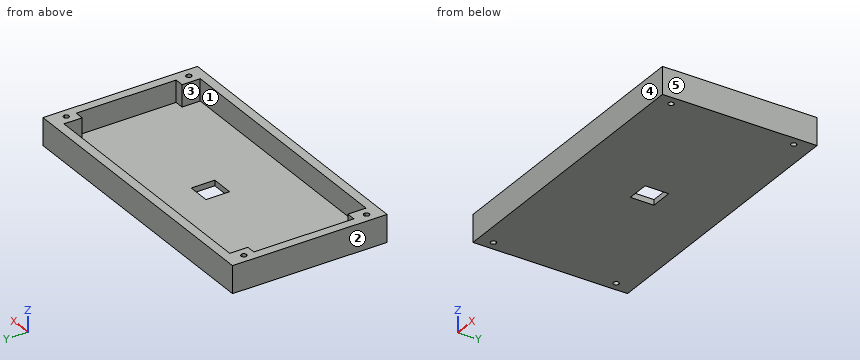
```python
from build123d import *

# Parameters (mm, degrees)
F0_W     = 160
F0_H     = 85
F0_W_2   = 12.5
F0_H_2   = 13
F1_DEPTH = 3
F2_W     = 160
F2_H     = 85
F2_W_2   = 150
F2_H_2   = 75
F3_DEPTH = 12
F5_DEPTH = 12
F6_DEPTH = 15


with BuildPart() as f1:
    # F0 (on Top) → F1 (new body)
    with BuildSketch(Plane.XY):
        with Locations((0, -2.5)):
            Rectangle(F0_W, F0_H)
        Rectangle(F0_W_2, F0_H_2, mode=Mode.SUBTRACT)
    extrude(amount=F1_DEPTH)

    # F2 (on face) → F3 (join)
    with BuildSketch(Plane.XY.offset(3)):
        with Locations((0, -2.5)):
            Rectangle(F2_W, F2_H)
        with Locations((0, -2.5)):
            Rectangle(F2_W_2, F2_H_2, mode=Mode.SUBTRACT)
    extrude(amount=F3_DEPTH)

    # F4 (on face) → F5 (join, through all)
    with BuildSketch(Plane.XY.offset(15)):
        with BuildLine():
            ThreePointArc((75, 29), (73.5, 30.5), (75, 32))
            Line((75, 32), (75, 35))
            Line((75, 35), (70, 35))
            Line((70, 35), (70, 25))
            Line((70, 25), (75, 25))
            Line((75, 25), (75, 29))
        make_face()
        with BuildLine():
            ThreePointArc((-75, 32), (-73.93934, 31.56066), (-73.5, 30.5))
            ThreePointArc((-73.5, 30.5), (-73.93934, 29.43934), (-75, 29))
            Line((-75, 29), (-75, 25))
            Line((-75, 25), (-70, 25))
            Line((-70, 25), (-70, 35))
            Line((-70, 35), (-75, 35))
            Line((-75, 35), (-75, 32))
        make_face()
        with BuildLine():
            ThreePointArc((-75, -35.5), (-73.93934, -35.93934), (-73.5, -37))
            ThreePointArc((-73.5, -37), (-73.93934, -38.06066), (-75, -38.5))
            Line((-75, -38.5), (-75, -40))
            Line((-75, -40), (-70, -40))
            Line((-70, -40), (-70, -30))
            Line((-70, -30), (-75, -30))
            Line((-75, -30), (-75, -35.5))
        make_face()
        with BuildLine():
            ThreePointArc((75, -38.5), (73.5, -37), (75, -35.5))
            Line((75, -35.5), (75, -30))
            Line((75, -30), (70, -30))
            Line((70, -30), (70, -40))
            Line((70, -40), (75, -40))
            Line((75, -40), (75, -38.5))
        make_face()
    extrude(amount=-F5_DEPTH)

    # F4 (on face) → F6 (cut, through all)
    with BuildSketch(Plane.XY.offset(15)):
        with BuildLine():
            ThreePointArc((-75, -38.5), (-73.93934, -38.06066), (-73.5, -37))
            ThreePointArc((-73.5, -37), (-73.93934, -35.93934), (-75, -35.5))
            Line((-75, -35.5), (-75, -38.5))
        make_face()
        with BuildLine():
            Line((-75, -38.5), (-75, -35.5))
            ThreePointArc((-75, -35.5), (-76.5, -37), (-75, -38.5))
        make_face()
        with BuildLine():
            ThreePointArc((75, -38.5), (76.06066, -38.06066), (76.5, -37))
            ThreePointArc((76.5, -37), (76.06066, -35.93934), (75, -35.5))
            Line((75, -35.5), (75, -38.5))
        make_face()
        with BuildLine():
            Line((75, -38.5), (75, -35.5))
            ThreePointArc((75, -35.5), (73.5, -37), (75, -38.5))
        make_face()
        with BuildLine():
            Line((75, 29), (75, 32))
            ThreePointArc((75, 32), (73.5, 30.5), (75, 29))
        make_face()
        with BuildLine():
            ThreePointArc((75, 29), (76.06066, 29.43934), (76.5, 30.5))
            ThreePointArc((76.5, 30.5), (76.06066, 31.56066), (75, 32))
            Line((75, 32), (75, 29))
        make_face()
        with BuildLine():
            ThreePointArc((-75, 29), (-73.93934, 29.43934), (-73.5, 30.5))
            ThreePointArc((-73.5, 30.5), (-73.93934, 31.56066), (-75, 32))
            Line((-75, 32), (-75, 29))
        make_face()
        with BuildLine():
            Line((-75, 29), (-75, 32))
            ThreePointArc((-75, 32), (-76.5, 30.5), (-75, 29))
        make_face()
    extrude(amount=-F6_DEPTH, mode=Mode.SUBTRACT)


solid = f1.part
```
Check sheet for the modelled part. Datum: model origin and axes. Units: mm. Face numbers are marked on the shaded views. A direction names the side the tool comes from. Round coordinates to 2 decimals unless told otherwise and drop trailing zeros. Write each loop counter-clockwise with the first axis right and the second up, starting at its lowest first coordinate (ties: lowest second). Pieces come first, ordered by that corner, then holes. Notation, with made-up numbers: (0, 18) -> (42, 18) arc R20 cw to (42, 40) -> close; hole circle Ø2 at (26.25, 48). An arc over 180 degrees is marked (long way). Put each result on its own line as item: value.
(1) Sectioned sample at B-B (x = -2). Enter the section's corners in (y, z).
Values found:
outline: (-45, 0) -> (-6.5, 0) -> (-6.5, 3) -> (-40, 3) -> (-40, 15) -> (-45, 15) -> close; (6.5, 0) -> (40, 0) -> (40, 15) -> (35, 15) -> (35, 3) -> (6.5, 3) -> close
(2) Material ranges on line 1 (Y direction, x = -31.5, z = 4.5); line 2 (X direction, y = 4, z = 10.5); line 3 (Y direction, x = 72.5, z = 8.5), recorded low to high.
Values found:
line 1: y = -45 to -40, 35 to 40
line 2: x = -80 to -75, 75 to 80
line 3: y = -45 to -30, 25 to 40
(3) Go/stop test with flat-tipped pins: pin 1 Ø2 at (x, y) = (-41.5, -23) entering from -Z; pin 2 Ø5 at (x, y) = (-31, 19) entering from +Z. Record where each tip stops, or that it passes through.
Values found:
pin 1: stops at z = 0
pin 2: stops at z = 3
(4) Mould release check, pull along Y, two halves, no side actions. Record for the marked faces 3, 4 and 5: released by +Y, released by -Y, zero draft, split by the parting line, or undercut.
Values found:
face 3: undercut
face 4: released by -Y
face 5: zero draft
(5) Sectioned sample at A-A (y = 2.5). Enter the section's corners in (x, z).
Values found:
outline: (-80, 0) -> (-6.25, 0) -> (-6.25, 3) -> (-75, 3) -> (-75, 15) -> (-80, 15) -> close; (6.25, 0) -> (80, 0) -> (80, 15) -> (75, 15) -> (75, 3) -> (6.25, 3) -> close
(6) Sectioned sample at D-D (x = 31). Enter the section's corners in (y, z).
Values found:
outline: (-45, 0) -> (40, 0) -> (40, 15) -> (35, 15) -> (35, 3) -> (-40, 3) -> (-40, 15) -> (-45, 15) -> close
(7) Tool access check on the marked faces 1 and 2. Record the directions out of +Z, -Z, +X, -X, +Y, -Y that give a thin tool (end or side, any length) a straight path to the whole face; none if there is none.
Values found:
face 1: +Z
face 2: +Z, -Z, -X, +Y, -Y
(8) Sectioned sample at C-C (z = 7.5). Enter the section's corners in (x, y), plus the area to 3 significant figures.
Values found:
outline: (-80, -45) -> (80, -45) -> (80, 40) -> (-80, 40) -> close; hole (-75, -35.5) arc R1.5 ccw (long way) to (-73.5, -37) arc R1.5 ccw to start; hole (-75, -30) -> (-70, -30) -> (-70, -40) -> (70, -40) -> (70, -30) -> (75, -30) -> (75, 25) -> (70, 25) -> (70, 35) -> (-70, 35) -> (-70, 25) -> (-75, 25) -> close; hole (-75, 32) arc R1.5 ccw (long way) to (-73.5, 30.5) arc R1.5 ccw to start; hole (75, -35.5) arc R1.5 ccw (long way) to (76.5, -37) arc R1.5 ccw to start; hole (75, 32) arc R1.5 ccw (long way) to (76.5, 30.5) arc R1.5 ccw to start
area: 2,520 mm^2
